Verification items for this drawing (mm, ordinates from the low corner). A direction names the side the tool comes from. Give positions to 0.01 mm unless a question says otherwise; leave off trailing zeros. Write each loop counter-clockwise with the first axis right and the second up, starting at its lowest first coordinate (ties: lowest second). Pieces come first, ordered by that corner, then holes. Notation, with made-up numbers: M -17,-17 L 32,-17 A18 cw 32,-7 Z; hole C 60.5,60.5 d10. An arc over 180 degrees is marked long. Write each question's results on one line, items separated by ' | '.
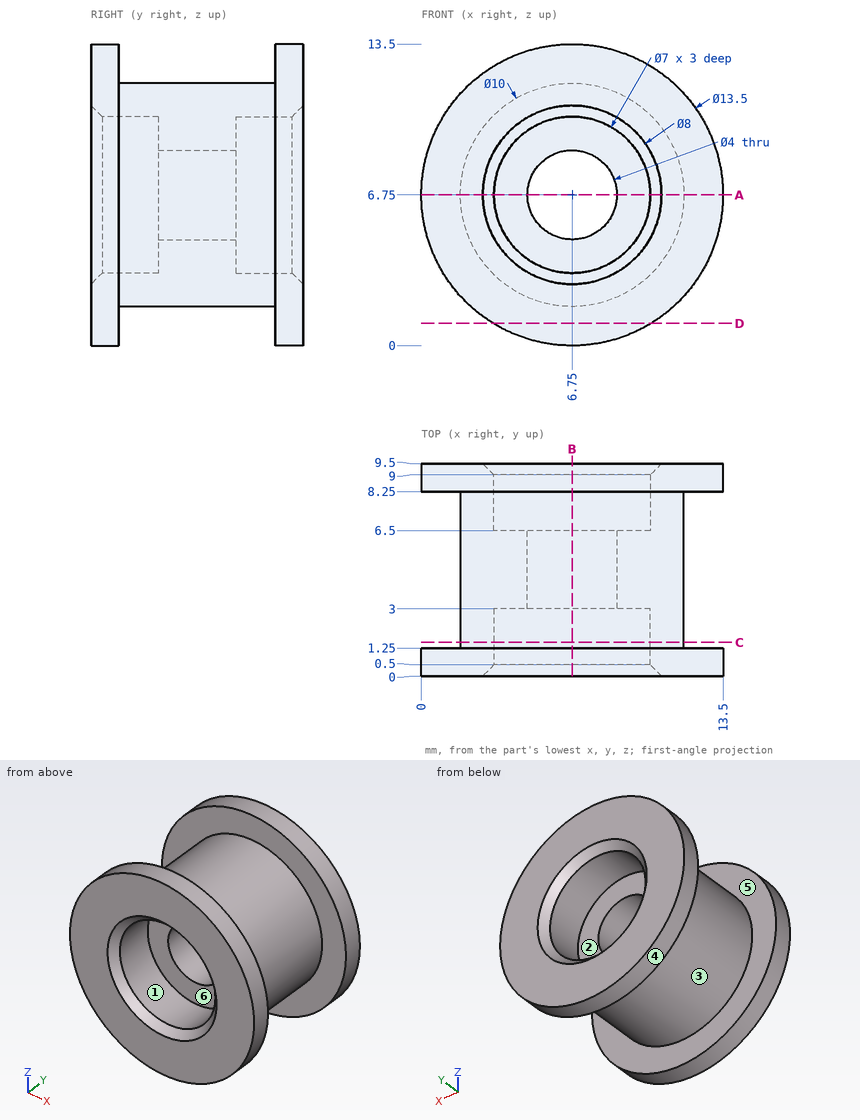
Q1. Section check C-C (y = 1.5). Enter the section's corners in (x, z).
Answer key:
outline: C 6.75,6.75 d10; hole C 6.75,6.75 d7
Q2. Access from +Z, -Z, +X, -X, +Y, -Y to the whole of each face (thin tool, end or side, straight path). Record for the marked faces 1, 2 and 3.
Answer key:
face 1: -Y | face 2: +Y | face 3: none
Q3. Material ranges on probe 1 along Z at (x, y) = (6.75, 5.5); probe 2 along Y at (x, z) = (12.75, 6.75), recorded low to high. Write a range as [from, to].
Answer key:
probe 1: z = [1.75, 4.75], [8.75, 11.75] | probe 2: y = [0, 1.25], [8.25, 9.5]
Q4. Section check D-D (z = 1). Enter the section's corners in (x, y).
Answer key:
outline: M 3.21,0 L 10.29,0 L 10.29,1.25 L 3.21,1.25 Z; M 3.21,8.25 L 10.29,8.25 L 10.29,9.5 L 3.21,9.5 Z
Q5. Depth check by flat-ended pin: P1, Ø2, axis at y = 4, z = 1.5, coming from the -X side; P2, Ø2, axis at x = 8.5, y = 7.5, coming from the -Z side; P3, Ø5, axis at x = 6.75, z = 6.75, coming from the +Y side. Enter the tip coordinate at first touch or a pass-through.
Answer key:
P1: stops at x = 4.12 | P2: stops at z = 0.09 | P3: stops at y = 6.5
Q6. Release check for a two-part mould opening along Z. For the marked faces 4, 5 and 6 record: released by +Z, released by -Z, zero draft, split by the parting line, or undercut.
Answer key:
face 4: split by the parting line | face 5: zero draft | face 6: undercut
Q7. Section check B-B (x = 6.75). Enter the section's corners in (y, z), then the cut area to 4 significant figures.
Answer key:
outline: M 0,0 L 1.25,0 L 1.25,1.75 L 8.25,1.75 L 8.25,0 L 9.5,0 L 9.5,2.75 L 9,3.25 L 6.5,3.25 L 6.5,4.75 L 3,4.75 L 3,3.25 L 0.5,3.25 L 0,2.75 Z; M 0,10.75 L 0.5,10.25 L 3,10.25 L 3,8.75 L 6.5,8.75 L 6.5,10.25 L 9,10.25 L 9.5,10.75 L 9.5,13.5 L 8.25,13.5 L 8.25,11.75 L 1.25,11.75 L 1.25,13.5 L 0,13.5 Z | area: 47.25 mm2
Q8. Section check A-A (z = 6.75). Enter the section's corners in (x, y), then the cut area to 4 significant figures.
Answer key:
outline: M 0,0 L 2.75,0 L 3.25,0.5 L 3.25,3 L 4.75,3 L 4.75,6.5 L 3.25,6.5 L 3.25,9 L 2.75,9.5 L 0,9.5 L 0,8.25 L 1.75,8.25 L 1.75,1.25 L 0,1.25 Z; M 8.75,3 L 10.25,3 L 10.25,0.5 L 10.75,0 L 13.5,0 L 13.5,1.25 L 11.75,1.25 L 11.75,8.25 L 13.5,8.25 L 13.5,9.5 L 10.75,9.5 L 10.25,9 L 10.25,6.5 L 8.75,6.5 Z | area: 47.25 mm2
